from build123d import *

# Parameters (mm, degrees)
F0_R     = 4.445
F1_DEPTH = 203.2
F2_W     = 61.176687
F2_H     = 14.94658
F2_R     = 2.485662
F3_DEPTH = 13.97
F4_R     = 2.54
F5_DEPTH = 25.4


with BuildPart() as f1:
    # F0 (on Top) → F1 (new body)
    with BuildSketch(Plane.XY):
        with Locations((-34.222286, 8.437074)):
            Circle(F0_R)
    extrude(amount=-F1_DEPTH)

    # F2 (on Front) → F3 (join)
    with BuildSketch(Plane.XZ):
        with Locations((-34.07263, -166.781291)):
            Rectangle(F2_W, F2_H)
        with Locations((-34.072631, -165.9123)):
            Circle(F2_R, mode=Mode.SUBTRACT)
    extrude(amount=-F3_DEPTH)

    # F4 (on face) → F5 (join)
    with BuildSketch(Plane(origin=(0, 13.97, 0), x_dir=(-1, 0, 0), z_dir=(0, 1, 0))):
        with Locations((34.072631, -165.9123)):
            Circle(F4_R)
    extrude(amount=-F5_DEPTH)


solid = f1.part
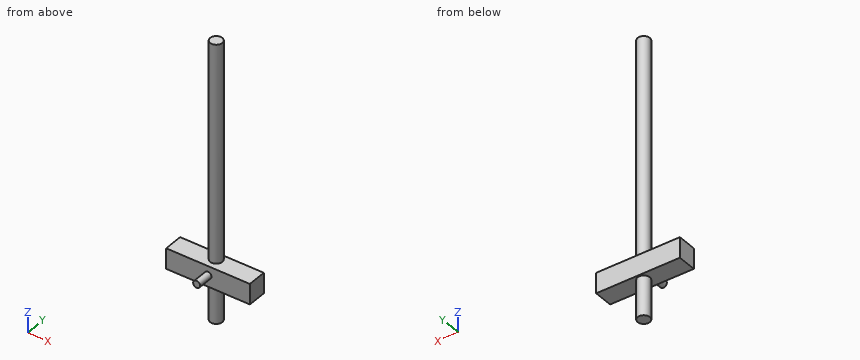
The model under review builds one solid part; all positions refer to its coordinate system, in mm. Round coordinates to 2 decimals unless told otherwise and drop trailing zeros. Write each loop counter-clockwise with the first axis right and the second up, starting at its lowest first coordinate (ties: lowest second). Pieces come first, ordered by that corner, then holes. Notation, with made-up numbers: (2.5, 20) - (18.5, 20) arc R18 cw to (18.5, 31) - close; hole circle Ø2 at (4.5, 14.5). An arc over 180 degrees is marked (long way). One line per item, written item: value. Start each with the question number.
1. Consider section D-D on x = -53.5. Write out the cut boundary in (y, z).
2. Consider section B-B on z = -70.5. Write out the cut boundary in (x, y) (3 decimals), and give its area (3 significant figures).
3. Consider section C-C on y = -9.25. Write out the cut boundary in (x, z).
4. Clearance check with flat-ended pins moving along their axes: P1, Ø4, axis at x = -46.5, y = 8, coming from the -Z side; P2, Ø7.5, axis at x = -23.5, z = -165.5, coming from the -Y side; P3, Ø3, axis at y = 3.5, z = -180.5, coming from the +X side; P4, Ø10, axis at x = -55, y = -5.5, coming from the +Z side. State where each tip first meets the part, or that it passes through.
5. Consider section A-A on x = -34. Write out the cut boundary in (y, z).
6. To check wall thickness, follow L1, parallel to Z at x = -12.5, y = 9.75; L2, parallel to Y at x = -8, z = -161.5; L3, parallel to Z at x = -34.5, y = -9.5. State the ranges of each line that lie inside material, in increasing order. Write a range as from..to.
Checks:
1. outline: (0, -174.25) - (13.97, -174.25) - (13.97, -159.31) - (0, -159.31) - close
2. outline: circle Ø8.89 at (-34.222, 8.437)
2. area: 62.1 mm^2
3. outline: circle Ø5.08 at (-34.07, -165.91)
4. P1: stops at z = -174.25
4. P2: stops at y = 0
4. P3: stops at x = -31.4
4. P4: passes through
5. outline: (-11.43, -168.45) - (0, -168.45) - (0, -174.25) - (4, -174.25) - (4, -203.2) - (12.88, -203.2) - (12.88, -174.25) - (13.97, -174.25) - (13.97, -159.31) - (12.88, -159.31) - (12.88, 0) - (4, 0) - (4, -159.31) - (0, -159.31) - (0, -163.37) - (-11.43, -163.37) - close
6. L1: z = -174.25..-159.31
6. L2: y = 0..13.97
6. L3: z = -168.42..-163.41
